```python
from build123d import *

# Parameters (mm, degrees)
F0_R     = 8.5
F0_R_2   = 8.3
F1_DEPTH = 20
F0_R_3   = 6
F2_DEPTH = 4
F3_R     = 2


with BuildPart() as f1:
    # F0 (on Top) → F1 (new body)
    with BuildSketch(Plane.XY):
        Circle(F0_R)
        Circle(F0_R_2, mode=Mode.SUBTRACT)
    extrude(amount=F1_DEPTH)

    # F0 (on Top) → F2 (join)
    with BuildSketch(Plane.XY):
        Circle(F0_R_2)
        Circle(F0_R_3, mode=Mode.SUBTRACT)
    extrude(amount=F2_DEPTH)

    # F3
    f3_edges = [f1.edges().sort_by_distance(p)[0] for p in [
        (-8.5, 0, 0),
    ]]
    fillet(f3_edges, radius=F3_R)


solid = f1.part
```
Geometry: final body of the model. Coordinates: model frame, mm. A direction names the side the tool comes from. Give positions to 0.01 mm unless a question says otherwise; leave off trailing zeros. Write each loop counter-clockwise with the first axis right and the second up, starting at its lowest first coordinate (ties: lowest second). Pieces come first, ordered by that corner, then holes.
1. Reachability of faces 1 (the cylindrical face through (-1.799, -8.103, 11.888)), 2 (the cylindrical face through (-6, 0, 2)) from +Z, -Z, +X, -X, +Y, -Y: full face, straight path, thin tool, end or side. Return the list, or none.
2. Section query A-A, the plane x = 0. Return loops of the section in (y, z), then the cut area to 3 significant figures.
3. Pin query (flat end, axial travel): P1, Ø8.5, axis at x = 0.5, y = 3.5, coming from the +Z side; P2, Ø4, axis at x = 4.5, z = 5, coming from the +Y side; P3, Ø1.5, axis at y = -4.5, z = 18, coming from the +X side. Return the tip coordinate at first contact, or that it passes through.
4. Line query: probe 1 along Y at (x, z) = (0, 12.75); probe 2 along Y at (x, z) = (0, 2.55); probe 3 along X at (y, z) = (7.5, 9.75). Output: solid intervals per line, ascending.
5. Draft query along Y for faces 3 (the flat face through (-2, 6, 4)), 4 (the cylindrical face through (4.57, 7.167, 10.874)), 5 (the flat face through (2, -6, 0)). Return one class per face: released by +Y, released by -Y, zero draft, split by the parting line, or undercut.
6. Section query C-C, the plane z = 17.5. Return loops of the section in (x, y), then the cut area to 3 significant figures.
Computed:
1. face 1: +Z
1. face 2: +Z, -Z
2. outline: (-8.5, 2) arc R2 ccw to (-6.5, 0) - (-6, 0) - (-6, 4) - (-8.3, 4) - (-8.3, 20) - (-8.5, 20) - close; (6, 0) - (6.5, 0) arc R2 ccw to (8.5, 2) - (8.5, 20) - (8.3, 20) - (8.3, 4) - (6, 4) - close
2. area: 24.7 mm2
3. P1: stops at z = 4
3. P2: stops at y = 8.12
3. P3: stops at x = 7.63
4. probe 1: y = -8.5 to -8.3, 8.3 to 8.5
4. probe 2: y = -8.5 to -6, 6 to 8.5
4. probe 3: x = -4 to -3.56, 3.56 to 4
5. face 3: undercut
5. face 4: split by the parting line
5. face 5: zero draft
6. outline: circle Ø17 at (0, 0); hole circle Ø16.6 at (0, 0)
6. area: 10.6 mm2
